```python
from build123d import *

# Parameters (mm, degrees)
SKETCH2_W           = 311.404
SKETCH2_H           = 311.404
BOSS_EXTRUDE1_DEPTH = 67.31
SKETCH4_W           = 289.56
SKETCH4_H           = 289.56
CUT_EXTRUDE1_DEPTH  = 25.4
SKETCH5_W           = 273.304
SKETCH5_H           = 273.304
CUT_EXTRUDE2_DEPTH  = 60.96
SKETCH6_W           = 304.8
SKETCH6_H           = 304.8
SKETCH6_W_2         = 298.196
SKETCH6_H_2         = 298.196
CUT_EXTRUDE3_DEPTH  = 12.7


with BuildPart() as part:
    # Sketch2 → Boss-Extrude1 (new body)
    with BuildSketch(Plane(origin=(0, 0, 0), x_dir=(1, 0, 0), z_dir=(0, 1, 0))):
        Rectangle(SKETCH2_W, SKETCH2_H)
    extrude(amount=BOSS_EXTRUDE1_DEPTH)

    # Sketch4 → Cut-Extrude1 (cut)
    with BuildSketch(Plane(origin=(0, 67.31, 0), x_dir=(1, 0, 0), z_dir=(0, 1, 0))):
        Rectangle(SKETCH4_W, SKETCH4_H)
    extrude(amount=-CUT_EXTRUDE1_DEPTH, mode=Mode.SUBTRACT)

    # Sketch5 → Cut-Extrude2 (cut)
    with BuildSketch(Plane(origin=(0, 67.31, 0), x_dir=(1, 0, 0), z_dir=(0, 1, 0))):
        Rectangle(SKETCH5_W, SKETCH5_H)
    extrude(amount=-CUT_EXTRUDE2_DEPTH, mode=Mode.SUBTRACT)

    # Sketch6 → Cut-Extrude3 (cut)
    with BuildSketch(Plane(origin=(0, 67.31, 0), x_dir=(1, 0, 0), z_dir=(0, 1, 0))):
        Rectangle(SKETCH6_W, SKETCH6_H)
        Rectangle(SKETCH6_W_2, SKETCH6_H_2, mode=Mode.SUBTRACT)
    extrude(amount=-CUT_EXTRUDE3_DEPTH, mode=Mode.SUBTRACT)


solid = part.part
```
Check sheet for the modelled part. Datum: model origin and axes. Units: mm. Give positions to 0.01 mm unless a question says otherwise; leave off trailing zeros. Write each loop counter-clockwise with the first axis right and the second up, starting at its lowest first coordinate (ties: lowest second). Pieces come first, ordered by that corner, then holes. Notation, with made-up numbers: (-14.75, 4) -> (18.25, 4) arc R16 ccw to (18.25, 21) -> close; hole circle Ø5 at (47.5, 0.5). An arc over 180 degrees is marked (long way). Use CSV: the item, a comma, the result in double quotes. Start each with the question number.
Q1. Release check for a two-part mould opening along Z. For faces 1 (the flat face through (-2, 33, -155.702)), 2 (the flat face through (-149.098, 61, 2)), 3 (the flat face through (-2, 24, -136.652)), 4 (the flat face through (155.702, 33, 2)) record: +Z half, -Z half, draft (parallel to the pull), parting line (faces both ways), or undercut.
Q2. Cross-section at A-A on y = 51. Enter the section's corners in (x, z), and give its area (3 significant figures).
Q3. Cross-section at C-C on x = -60.5. Enter the section's corners in (y, z), and give its area (3 significant figures).
Q4. Scan lines: line 1 along Z through (x, y) = (-5, 63); line 2 along Z through (x, y) = (87, 11.5). Record each from-to range of solid material in increasing order.
Q5. Cross-section at B-B on z = -82. Enter the section's corners in (x, y).
Q6. Depth check by flat-ended pin: P1, Ø5, axis at x = 10.5, z = 8.5, coming from the +Y side. Enter the tip coordinate at first touch or a pass-through.
Q7. Cross-section at D-D on y = 35. Enter the section's corners in (x, z), and give its area (3 significant figures).
Working result:
1,face 1,"-Z half"
1,face 2,"undercut"
1,face 3,"undercut"
1,face 4,"draft"
2,outline,"(-155.7, -155.7) -> (155.7, -155.7) -> (155.7, 155.7) -> (-155.7, 155.7) -> close; hole (-144.78, -144.78) -> (144.78, -144.78) -> (144.78, 144.78) -> (-144.78, 144.78) -> close"
2,area,"13,100 mm^2"
3,outline,"(0, -155.7) -> (67.31, -155.7) -> (67.31, -152.4) -> (54.61, -152.4) -> (54.61, -149.1) -> (67.31, -149.1) -> (67.31, -144.78) -> (41.91, -144.78) -> (41.91, -136.65) -> (6.35, -136.65) -> (6.35, 136.65) -> (41.91, 136.65) -> (41.91, 144.78) -> (67.31, 144.78) -> (67.31, 149.1) -> (54.61, 149.1) -> (54.61, 152.4) -> (67.31, 152.4) -> (67.31, 155.7) -> (0, 155.7) -> close"
3,area,"3,800 mm^2"
4,line 1,"z = -155.7 to -152.4, -149.1 to -144.78, 144.78 to 149.1, 152.4 to 155.7"
4,line 2,"z = -155.7 to -136.65, 136.65 to 155.7"
5,outline,"(-155.7, 0) -> (155.7, 0) -> (155.7, 67.31) -> (152.4, 67.31) -> (152.4, 54.61) -> (149.1, 54.61) -> (149.1, 67.31) -> (144.78, 67.31) -> (144.78, 41.91) -> (136.65, 41.91) -> (136.65, 6.35) -> (-136.65, 6.35) -> (-136.65, 41.91) -> (-144.78, 41.91) -> (-144.78, 67.31) -> (-149.1, 67.31) -> (-149.1, 54.61) -> (-152.4, 54.61) -> (-152.4, 67.31) -> (-155.7, 67.31) -> close"
6,P1,"stops at y = 6.35"
7,outline,"(-155.7, -155.7) -> (155.7, -155.7) -> (155.7, 155.7) -> (-155.7, 155.7) -> close; hole (-136.65, -136.65) -> (136.65, -136.65) -> (136.65, 136.65) -> (-136.65, 136.65) -> close"
7,area,"22,300 mm^2"
